Geometry: final body of the model. Coordinates: model frame, mm. Give positions to 0.01 mm unless a question says otherwise; leave off trailing zeros. Write each loop counter-clockwise with the first axis right and the second up, starting at its lowest first coordinate (ties: lowest second). Pieces come first, ordered by that corner, then holes. Notation, with made-up numbers: M -10.5,42 L 16.5,42 A11 cw 16.5,48 Z; hole C 37.5,15.25 d8. An arc over 180 degrees is marked long. Use a Markdown table: item, result. Add a question column.
1) Section A-A on z = 11. Return the cut outline in (x, y).
2) Line query: line 1 (Z direction, x = -10.25, y = -11); line 2 (X direction, y = 11.5, z = -11.5); line 3 (Z direction, x = 11.75, y = 2). Output: solid intervals per line, ascending.
3) Section B-B on y = -7. Return the cut outline in (x, z), then the cut area to 3 significant figures.
```python
from build123d import *

# Parameters (mm, degrees)
F0_W     = 25
F0_H     = 25
F1_DEPTH = 12.5


with BuildPart() as f1:
    # F0 (on Front) → F1 (new body, symmetric)
    with BuildSketch(Plane.XZ):
        Rectangle(F0_W, F0_H)
    extrude(amount=F1_DEPTH, both=True)

    # F2 (on Front) → F3 (revolve, intersect)
    with BuildSketch(Plane.XZ):
        with BuildLine():
            Line((0, -17.155538), (0, 17.155538))
            ThreePointArc((0, 17.155538), (-17.155538, 0), (0, -17.155538))
        make_face()
    revolve(axis=Axis((0, 0, 0), (0, 0, -1)), mode=Mode.INTERSECT)


solid = f1.part
```
Found:
| question | item | result |
|---|---|---|
| 1 | outline | M -12.5,-4.13 A13.16 ccw -4.13,-12.5 L 4.13,-12.5 A13.16 ccw 12.5,-4.13 L 12.5,4.13 A13.16 ccw 4.13,12.5 L -4.13,12.5 A13.16 ccw -12.5,4.13 Z |
| 2 | line 1 | -8.26 to 8.26 |
| 2 | line 2 | -5.46 to 5.46 |
| 2 | line 3 | -12.34 to 12.34 |
| 3 | outline | M -12.5,-9.44 A15.66 ccw -9.44,-12.5 L 9.44,-12.5 A15.66 ccw 12.5,-9.44 L 12.5,9.44 A15.66 ccw 9.44,12.5 L -9.44,12.5 A15.66 ccw -12.5,9.44 Z |
| 3 | area | 608 mm² |
